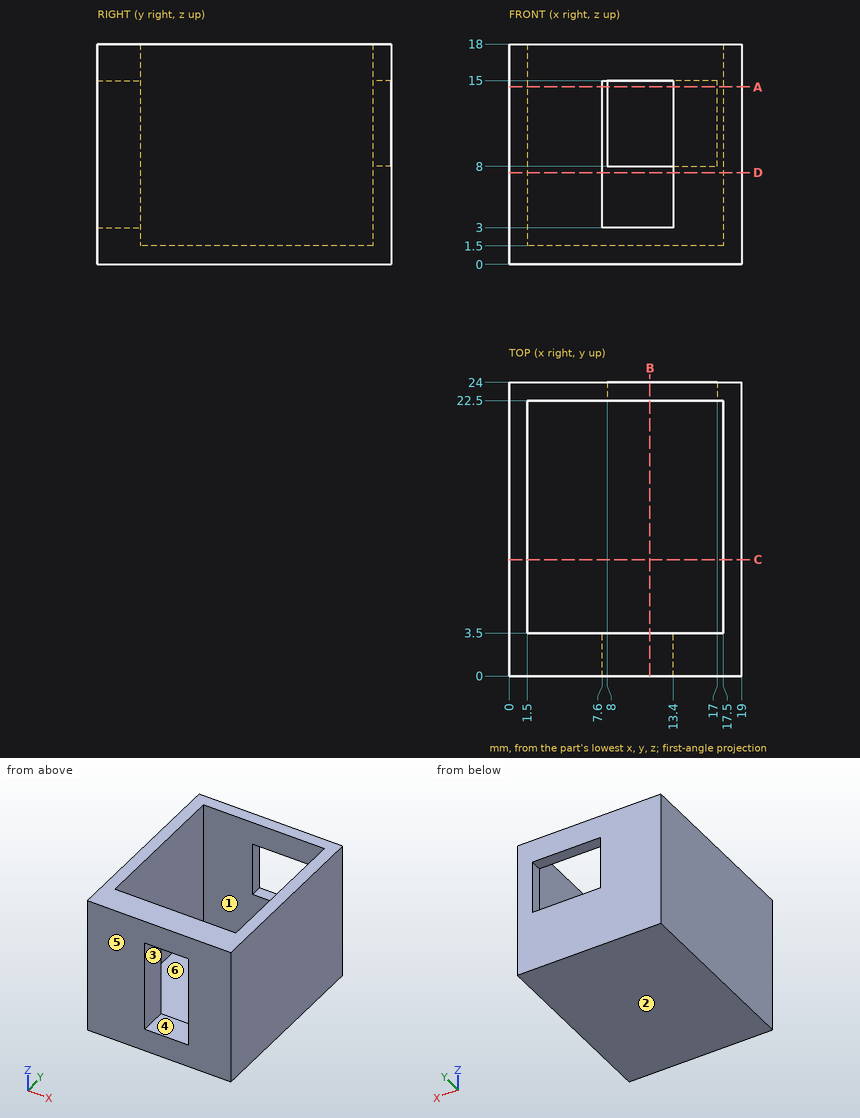
Here's the drawing with two shaded views (mm, measured from the low corner). I have some questions. A direction names the side the tool comes from. Give positions to 0.01 mm unless a question says otherwise; leave off trailing zeros. Loops run counter-clockwise (first coordinate to the right, second up) from the corner with the lowest first, then second, coordinate; pieces in that order, holes last. Notation, with made-up numbers: M -32.75,42.5 L -16.75,42.5 A12 ccw -16.75,49.5 Z; hole C 22.5,-20.5 d10. An arc over 180 degrees is marked long. One line per item, written item: value. Start each with the question number.
1) Thinking about a two-plate mould opening in Z: for the marked faces 4, 5 and 6, which applies, +Z half, -Z half, draft (parallel to the pull), parting line (faces both ways), or undercut?
2) I'm going to push a flat-ended pin straight in: pin 1 (8 mm diameter, centred on x = 7.5, y = 8.5, fed in from +Z). Where does the tip first touch, or does it pass through?
3) If we section it at B-B, the plane x = 11.5: Write out the boundary of the cut face in (y, z).
4) On a 3-axis mill with a long thin cutter (end or side, diameter ignored), from which of +Z, -Z, +X, -X, +Y, -Y can I reach the whole of each face in a straight line? I mean the marked faces 1, 2 and 3. Say none if no direction works.
5) If we section it at A-A, the plane z = 14.5: Write out the boundary of the cut face in (x, y).
6) If we section it at D-D, the plane z = 7.5: Write out the boundary of the cut face in (x, y).
7) If I drill on line 1 (Y direction, x = 7.5, z = 10.25); line 2 (X direction, y = 20.5, z = 5.75); line 3 (X direction, y = 3.25, z = 12.5), over which ranges is the centre line in solid material (lowest first)? Write a range as [from, to].
8) If we section it at C-C, the plane y = 9.5: Write out the boundary of the cut face in (x, z).
Completed:
1. face 4: undercut
1. face 5: draft
1. face 6: +Z half
2. pin 1: stops at z = 1.5
3. outline: M 0,0 L 24,0 L 24,8 L 22.5,8 L 22.5,1.5 L 3.5,1.5 L 3.5,3 L 0,3 Z; M 0,15 L 3.5,15 L 3.5,18 L 0,18 Z; M 22.5,15 L 24,15 L 24,18 L 22.5,18 Z
4. face 1: +Z
4. face 2: -Z, +X, -X, +Y, -Y
4. face 3: -Y
5. outline: M 0,0 L 7.6,0 L 7.6,3.5 L 1.5,3.5 L 1.5,22.5 L 8,22.5 L 8,24 L 0,24 Z; M 13.4,0 L 19,0 L 19,24 L 17,24 L 17,22.5 L 17.5,22.5 L 17.5,3.5 L 13.4,3.5 Z
6. outline: M 0,0 L 7.6,0 L 7.6,3.5 L 1.5,3.5 L 1.5,22.5 L 17.5,22.5 L 17.5,3.5 L 13.4,3.5 L 13.4,0 L 19,0 L 19,24 L 0,24 Z
7. line 1: y = [0, 3.5], [22.5, 24]
7. line 2: x = [0, 1.5], [17.5, 19]
7. line 3: x = [0, 7.6], [13.4, 19]
8. outline: M 0,0 L 19,0 L 19,18 L 17.5,18 L 17.5,1.5 L 1.5,1.5 L 1.5,18 L 0,18 Z
